from build123d import *

# Parameters (mm, degrees)
F1_DEPTH = 10
F2_DEPTH = 6.3
F3_R     = 1.65
F4_DEPTH = 25


with BuildPart() as f1:
    # F0 (on Top) → F1 (new body)
    with BuildSketch(Plane.XY):
        with BuildLine():
            ThreePointArc((4.5, 0), (12.5, 8), (20.5, 0))
            Line((20.5, 0), (25, 0))
            Line((25, 0), (25, 15))
            Line((25, 15), (0, 15))
            Line((0, 15), (0, 0))
            Line((0, 0), (4.5, 0))
        make_face()
    extrude(amount=F1_DEPTH)

    # F0 (on Top) → F2 (join)
    with BuildSketch(Plane.XY):
        with BuildLine():
            ThreePointArc((6.5, 0), (12.5, 6), (18.5, 0))
            Line((18.5, 0), (20.5, 0))
            ThreePointArc((20.5, 0), (12.5, 8), (4.5, 0))
            Line((4.5, 0), (6.5, 0))
        make_face()
    extrude(amount=F2_DEPTH)

    # F3 (on face) → F4 (cut)
    with BuildSketch(Plane(origin=(0, 15, 0), x_dir=(-1, 0, 0), z_dir=(0, 1, 0))):
        with Locations((-22.75, 5)):
            Circle(F3_R)
        with BuildLine():
            ThreePointArc((-0.6, 5), (-2.25, 6.65), (-3.9, 5))
            ThreePointArc((-3.9, 5), (-2.25, 3.35), (-0.6, 5))
        make_face()
    extrude(amount=-F4_DEPTH, mode=Mode.SUBTRACT)


solid = f1.part
Geometry: final body of the model. Coordinates: model frame, mm. Round coordinates to 2 decimals unless told otherwise and drop trailing zeros. Loops run counter-clockwise (first coordinate to the right, second up) from the corner with the lowest first, then second, coordinate; pieces in that order, holes last.
Q1. Section D-D on y = 12.5. Return loops of the section in (x, z).
Q2. Pin query (flat end, axial travel): P1, Ø5.5, axis at x = 2.25, z = 5, coming from the +Y side; P2, Ø6, axis at x = 10, y = 4, coming from the +Z side; P3, Ø2, axis at x = 13.5, z = 6, coming from the -Y side. Return the tip coordinate at first contact, or that it passes through.
Q3. Section C-C on z = 5. Return loops of the section in (x, y), plus the area to 3 significant figures.
Q4. Section A-A on x = 22.75. Return loops of the section in (y, z).
Q5. Pull-direction query (X, two-part tool) for faces 1 (the flat face through (25, 7, 5)), 2 (the flat face through (21, 0, 4)), 3 (the flat face through (12, 7, 6.3)), 4 (the cylindrical face through (12.324, 7.998, 8.124)); classes: released by +X, released by -X, zero draft, split by the parting line, or undercut.
Q6. Material intervals for L1, parallel to X at y = 8.25, z = 4; L2, parallel to X at y = 10.5, z = 3.5; L3, parallel to Z at x = 22.75, y = 11, sorted ascending.
Q7. Section B-B on y = 2.25. Return loops of the section in (x, z), plus the area to 3 significant figures.
Evaluation:
1. outline: (0, 0) - (25, 0) - (25, 10) - (0, 10) - close; hole circle Ø3.3 at (2.25, 5); hole circle Ø3.3 at (22.75, 5)
2. P1: stops at y = 15
2. P2: stops at z = 6.3
2. P3: stops at y = 5.66
3. outline: (0, 0) - (0.6, 0) - (0.6, 15) - (0, 15) - close; (3.9, 0) - (6.5, 0) arc R6 cw to (18.5, 0) - (21.1, 0) - (21.1, 15) - (3.9, 15) - close; (24.4, 0) - (25, 0) - (25, 15) - (24.4, 15) - close
3. area: 219 mm2
4. outline: (0, 0) - (15, 0) - (15, 3.35) - (0, 3.35) - close; (0, 6.65) - (15, 6.65) - (15, 10) - (0, 10) - close
5. face 1: released by +X
5. face 2: zero draft
5. face 3: undercut
5. face 4: undercut
6. L1: x = 0 to 0.94, 3.56 to 21.44, 24.06 to 25
6. L2: x = 0 to 1.56, 2.94 to 22.06, 23.44 to 25
6. L3: z = 0 to 3.35, 6.65 to 10
7. outline: (0, 0) - (6.94, 0) - (6.94, 6.3) - (4.82, 6.3) - (4.82, 10) - (0, 10) - close; (18.06, 0) - (25, 0) - (25, 10) - (20.18, 10) - (20.18, 6.3) - (18.06, 6.3) - close; hole circle Ø3.3 at (2.25, 5); hole circle Ø3.3 at (22.75, 5)
7. area: 106 mm2
